Geometry: see drawing. Coordinates: mm, zero at the bounding-box minimum. A direction names the side the tool comes from. Give positions to 0.01 mm unless a question says otherwise; leave off trailing zeros. Loops run counter-clockwise (first coordinate to the right, second up) from the corner with the lowest first, then second, coordinate; pieces in that order, holes last. Notation, with made-up numbers: M -6,-12 L 50,-12 A17 cw 50,5 Z; hole C 14,-11 d3. An arc over 180 degrees is marked long. Use CSV: the item, a comma, the result in double quotes. Start each with the question number.
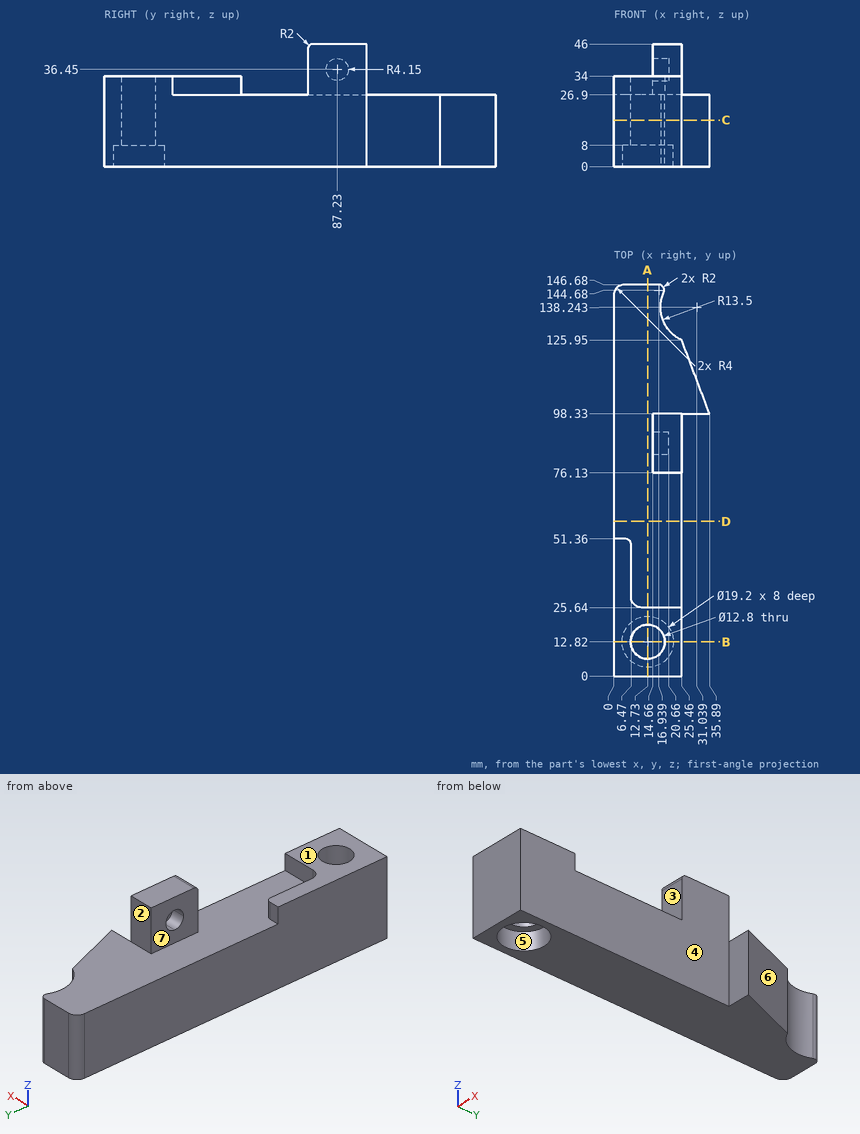
Item 1: Section D-D (y = 58). Output: boundary loops of the cut face in (x, z).
Item 2: Section C-C (z = 17.5). Output: boundary loops of the cut face in (x, y).
Item 3: Set-up query: the marked faces 1, 2, 3 and 4. Return all of +Z, -Z, +X, -X, +Y, -Y with unobstructed straight access to the full face (end or side cutting, diameter ignored); none if empty.
Item 4: Mould query, pull axis Y, two halves, no side actions, for the marked faces 5, 6 and 7. Classes: +Y half, -Y half, draft (parallel to the pull), parting line (faces both ways), or undercut.
Item 5: Material intervals for line 1 (Y direction, x = 12.5, z = 16); line 2 (Y direction, x = 16.5, z = 27); line 3 (X direction, y = 12.82, z = 25), sorted ascending.
Item 6: Section B-B (y = 12.82). Output: boundary loops of the cut face in (x, z).
Item 7: Section A-A (x = 12.73). Output: boundary loops of the cut face in (y, z), then the cut area to 3 significant figures.
Item 8: First-contact query: pin 1 Ø5 at (x, z) = (28, 12.5) entering from -Y; pin 2 Ø2 at (y, z) = (44, 29) entering from +X; pin 3 Ø9 at (y, z) = (88.5, 38) entering from -X. Flat tips, straight axial feed; report the tip coordinate or a pass-through.
Recorded:
1,outline,"M 0,0 L 25.46,0 L 25.46,26.9 L 0,26.9 Z"
2,outline,"M 0,0 L 25.46,0 L 25.46,98.33 L 35.89,98.33 L 25.46,125.95 A13.5 cw 18.76,143.85 A2 ccw 16.94,146.68 L 4,146.68 A4 ccw 0,142.68 Z; hole C 12.73,12.82 d12.8"
3,face 1,"+Z, +X, -X, -Y"
3,face 2,"+Z, +X, -X, +Y"
3,face 3,"+Z, +X, -X"
3,face 4,"+Z, -Z, +X, -Y"
4,face 5,"undercut"
4,face 6,"+Y half"
4,face 7,"draft"
5,line 1,"0 to 6.42, 19.22 to 146.68"
5,line 2,"0 to 7.65, 17.99 to 25.64, 76.13 to 98.33"
5,line 3,"0 to 6.33, 19.13 to 25.46"
6,outline,"M 0,0 L 3.13,0 L 3.13,8 L 6.33,8 L 6.33,34 L 0,34 Z; M 19.13,8 L 22.33,8 L 22.33,0 L 25.46,0 L 25.46,34 L 19.13,34 Z"
7,outline,"M 0,0 L 3.22,0 L 3.22,8 L 6.42,8 L 6.42,34 L 0,34 Z; M 19.22,8 L 22.42,8 L 22.42,0 L 146.68,0 L 146.68,26.9 L 25.64,26.9 L 25.64,34 L 19.22,34 Z"
7,area,"3,640 mm²"
8,pin 1,"y = 98.33"
8,pin 2,"x = 6.47"
8,pin 3,"x = 14.66"
